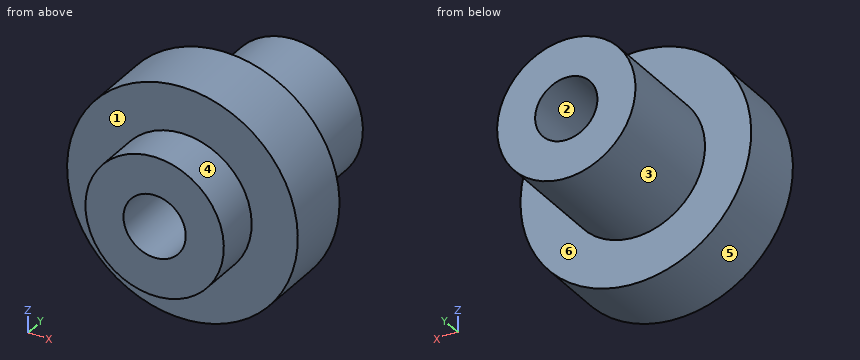
from build123d import *

# Parameters (mm, degrees)
HOLE_WIZARD_2_7_2_7_1_D = 2.7


with BuildPart() as part:
    # 草圖1 → 旋轉1 (revolve)
    with BuildSketch(Plane(origin=(0, 0, 0), x_dir=(0, 0, -1), z_dir=(1, 0, 0)), mode=Mode.PRIVATE) as revolve_1_sk:
        Polygon((0, 0), (3, 0), (3, 2), (5, 2), (5, 5), (3, 5), (3, 10), (0, 10), align=None)
    revolve(revolve_1_sk.sketch.rotate(Axis((0, 10, 0), (0, -1, 0)), 180), axis=Axis((0, 10, 0), (0, -1, 0)))

    # Ø2.7 (2.7) 直徑孔1 (through all)
    with Locations(Plane(origin=(0, 10, 0), x_dir=(1, 0, 0), z_dir=(0, 1, 0))):
        with Locations((0, 0)):
            Hole(HOLE_WIZARD_2_7_2_7_1_D / 2)


solid = part.part
Could you check a few things on this model? Use its own coordinates, in mm. Face numbers are marked on the shaded views. A direction names the side the tool comes from. Give positions to 0.01 mm unless a question says otherwise; leave off trailing zeros. Order: outer loops, then holes, each group sorted by start corner. A loop starts at its lowest first (then second) coordinate and runs counter-clockwise, first axis right, second up.
Item 1: For the marked faces 4, 5 and 6, which set-ups out of +Z, -Z, +X, -X, +Y, -Y let a thin tool reach every point of the face, with its end or its side?
Item 2: If we section it at D-D, the plane x = 4.75: Write out the boundary of the cut face in (y, z), plus the area to 3 significant figures.
Item 3: I need wall thicknesses on line 1 (Y direction, x = 0.75, z = 4); line 2 (Z direction, x = 1, y = 0.5); line 3 (X direction, y = 6.75, z = 0.25). Which ranges of each line are inside material? Lowest first, please.
Item 4: If we section it at C-C, the plane z = 2.5: Write out the boundary of the cut face in (x, y).
Item 5: If we mould it in two halves opening along X, with no side actions, what happens to the marked faces 1, 2 and 3? For each: pulls with the +X half, pulls with the -X half, needs draft (parallel to the pull), parting line crosses it, or undercut.
Item 6: If we section it at A-A, the plane x = 0: Write out the boundary of the cut face in (y, z).
Item 7: If we section it at B-B, the plane z = 1: Write out the boundary of the cut face in (x, y), plus the area to 3 significant figures.
Item 8: I'm going to push flat-ended pins straight in: pin 1 (1.5 mm diameter, centred on x = 2, y = 6, fed in from -Z); pin 2 (4 mm diameter, centred on x = -2, z = 3.5, fed in from +Y); pin 3 (1.5 mm diameter, centred on y = 2.5, z = 3.5, fed in from -X). Where does each tip first touch, or does it pass through?
Values:
1. face 4: -Y
1. face 5: +Y, -Y
1. face 6: +Y
2. outline: (2, -1.56) - (5, -1.56) - (5, 1.56) - (2, 1.56) - close
2. area: 9.37 mm2
3. line 1: y = 2 to 5
3. line 2: z = -2.83 to -0.91, 0.91 to 2.83
3. line 3: x = -2.99 to -1.33, 1.33 to 2.99
4. outline: (-4.33, 2) - (-1.66, 2) - (-1.66, 0) - (1.66, 0) - (1.66, 2) - (4.33, 2) - (4.33, 5) - (1.66, 5) - (1.66, 10) - (-1.66, 10) - (-1.66, 5) - (-4.33, 5) - close
5. face 1: needs draft
5. face 2: undercut
5. face 3: parting line crosses it
6. outline: (0, -3) - (2, -3) - (2, -5) - (5, -5) - (5, -3) - (10, -3) - (10, -1.35) - (0, -1.35) - close; (0, 1.35) - (10, 1.35) - (10, 3) - (5, 3) - (5, 5) - (2, 5) - (2, 3) - (0, 3) - close
7. outline: (-4.9, 2) - (-2.83, 2) - (-2.83, 0) - (-0.91, 0) - (-0.91, 10) - (-2.83, 10) - (-2.83, 5) - (-4.9, 5) - close; (0.91, 0) - (2.83, 0) - (2.83, 2) - (4.9, 2) - (4.9, 5) - (2.83, 5) - (2.83, 10) - (0.91, 10) - close
7. area: 50.9 mm2
8. pin 1: stops at z = -2.73
8. pin 2: stops at y = 10
8. pin 3: stops at x = -4.18
